from build123d import *

# Parameters (mm, degrees)
EXTRUDE_2_DEPTH = 7.5


with BuildPart() as part:
    # 草图1 → 旋转1 (revolve)
    with BuildSketch(Plane.XY):
        Polygon((-5, 0), (0, 0), (20.5, 0), (20.5, 4.5), (10, 4.5), (10, 5), (0, 5), (0, 6.5), (-5, 6.5), (-5, 5), align=None)
    revolve(axis=Axis((-5, 0, 0), (1, 0, 0)))

    # 草图3 → 切除-旋转1 (revolve, cut)
    with BuildSketch(Plane(origin=(17.5, 0, 0), x_dir=(0, 0, -1), z_dir=(1, 0, 0))):
        Polygon((-6.680542038, 0), (-6.680542038, 1.407519777), (7.599960071, 1.407519777), (7.599960071, -0.067480223), align=None)
    revolve(axis=Axis((17.5, 0, 6.680542038), (0, -0.004725287, -0.999988836)), mode=Mode.SUBTRACT)

    # 草图4 → 凸台-拉伸2 (add)
    with BuildSketch(Plane.ZY.offset(5)):
        with BuildLine():
            Line((0.04652715, 0.75), (0, 0.75))
            Line((0, 0.75), (-1.58113883, 0.75))
            ThreePointArc((-1.58113883, 0.75), (0, -1.75), (1.58113883, 0.75))
            Line((1.58113883, 0.75), (0.04652715, 0.75))
        make_face()
    extrude(amount=EXTRUDE_2_DEPTH)


solid = part.part
Check sheet for the modelled part. Datum: model origin and axes. Units: mm. A direction names the side the tool comes from. Round coordinates to 2 decimals unless told otherwise and drop trailing zeros. Order: outer loops, then holes, each group sorted by start corner. A loop starts at its lowest first (then second) coordinate and runs counter-clockwise, first axis right, second up.
(1) Cross-section at B-B, the plane x = -0.5. Enter the section's corners in (y, z).
(2) Go/stop test with flat-tipped pins: P1, Ø1.5, axis at y = 0.5, z = -3, coming from the -X side; P2, Ø6, axis at x = 10.5, y = 2.5, coming from the -Z side; P3, Ø5, axis at x = -8.5, y = -1.5, coming from the -Z side. Record where each tip stops, or that it passes through.
(3) Cross-section at D-D, the plane x = -6.5. Enter the section's corners in (y, z).
(4) Cross-section at A-A, the plane x = 8.5. Enter the section's corners in (y, z).
(5) Access from +Z, -Z, +X, -X, +Y, -Y to the whole of each face (thin tool, end or side, straight path). Record for faces 4 (the flat face through (-9, 0.75, 0)), 5 (the cylindrical face through (15.18, 2.08, -3.99)), 6 (the flat face through (20.5, 0, 0)).
(6) Draft check along X on faces 1 (the cylindrical face through (-8.7, -1.75, -0.05)), 2 (the flat face through (-12.5, 0, 0)), 3 (the conical face through (18.714, 0.742, -0.067)). Enter one of: pulls with the +X half, pulls with the -X half, needs draft (parallel to the pull), parting line crosses it, or undercut.
(7) Scan lines: probe 1 along X at (y, z) = (3, 5.25); probe 2 along X at (y, z) = (-4.25, -1.25); probe 3 along Y at (x, z) = (18.5, -3.25). Record each from-to range of solid material in increasing order.
(8) Cross-section at C-C, the plane z = 5.5. Enter the section's corners in (x, y), and give its area (3 significant figures).
Check sheet entries:
1. outline: circle Ø13 at (0, 0)
2. P1: stops at x = -5
2. P2: stops at z = -5
2. P3: stops at z = -1.75
3. outline: (0.75, -1.58) - (0.75, 1.58) arc R1.75 ccw (long way) to start
4. outline: circle Ø10 at (0, 0)
5. face 4: +Z, -Z, -X, +Y
5. face 5: +X
5. face 6: +Z, -Z, +X, +Y, -Y
6. face 1: needs draft
6. face 2: pulls with the -X half
6. face 3: undercut
7. probe 1: x = -5 to 0
7. probe 2: x = -5 to 20.5
7. probe 3: y = -3.11 to -1.1, 1.01 to 3.11
8. outline: (-5, -3.46) - (0, -3.46) - (0, 3.46) - (-5, 3.46) - close
8. area: 34.6 mm2
